Autodesk Inventor part; units mm, degrees
ref_plane "YZ Plane" through (0, 0, 0) normal (1, 0, 0) x (0, 1, 0)
ref_plane "XZ Plane" through (0, 0, 0) normal (0, 1, 0) x (-1, 0, 0)
ref_plane "XY Plane" through (0, 0, 0) normal (0, 0, 1) x (1, 0, 0)
sketch "Sketch1" plane through (0, 0, 0) normal (0, 1, 0) x (-1, 0, 0)
  circle A0 centre (0, 0) radius 4
  circle A1 centre (0, 0) radius 35
  circle A2 centre (0, -28) radius 2
  circle A3 centre (14, -24.2487) radius 2
  circle A4 centre (24.2487, -14) radius 2
  circle A5 centre (28, 0) radius 2
  circle A6 centre (24.2487, 14) radius 2
  circle A7 centre (14, 24.2487) radius 2
  circle A8 centre (0, 28) radius 2
  circle A9 centre (-14, 24.2487) radius 2
  circle A10 centre (-24.2487, 14) radius 2
  circle A11 centre (-28, 0) radius 2
  circle A12 centre (-24.2487, -14) radius 2
  circle A13 centre (-14, -24.2487) radius 2
  circle A14 centre (-12, 0) radius 2.05
  circle A15 centre (6, -10.3923) radius 2.05
  circle A16 centre (6, 10.3923) radius 2.05
  dimension "d0" = 70
  dimension "d1" = 8
  dimension "d4" = 4
  dimension "d5" = 28
  dimension "d8" = 360
  dimension "d21" = 14.4939
  dimension "d53" = 12
  dimension "d54" = 4.1
  dimension "d57" = 360
extrude "Extrusion1" add sketch "Sketch1" along normal blind 4 contours A1 | A2 | A3 | A4 | A5 | A6 | A7 | A8 | A9 | A10 | A11 | A12 | A13
chamfer "Chamfer2" distance 0.5 angle 45 4 edges at (35, 4, 0) (4, 4, 0) (35, 0, 0) (4, 0, 0)
chamfer "Chamfer3" distance 2.5 angle 45 3 edges at (-3.95, 4, 10.3923) (-3.95, 4, -10.3923) (14.05, 4, 0)
hole "Hole1" at (-24.2487, 0, -14) at (-28, 0, 0) at (-24.2487, 0, 14) at (-14, 0, 24.2487) at (0, 0, 28) at (14, 0, 24.2487) at (24.2487, 0, 14) at (28, 0, 0) at (24.2487, 0, -14) at (14, 0, -24.2487) at (0, 0, -28) at (-14, 0, -24.2487) direction (0, 1, 0) diameter 3.242 depth 15 tip angle 118
properties part number "end effector mount 4 mm" material "Aluminum 6061"
The model under review builds one solid part; all positions refer to its coordinate system, in mm. Coordinates: 2 decimals unless noted, no trailing zeros. Order: outer loops, then holes, each group sorted by start corner. A loop starts at its lowest first (then second) coordinate and runs counter-clockwise, first axis right, second up. Notation, with made-up numbers: (22.5, 0.25) -> (36.5, 0.25) arc R8 cw to (36.5, 4.25) -> close; hole circle Ø11 at (-34.5, -29). An arc over 180 degrees is marked (long way). Answer in a Markdown table with one row per item. Add a question column.
Item 1: Clearance check with flat-ended pins moving along their axes: pin 1 (1.9 mm diameter, centred on x = 0, z = 28, fed in from +Y); pin 2 (1.5 mm diameter, centred on y = 1, z = -15, fed in from -X); pin 3 (2 mm diameter, centred on x = -23.5, y = 1.5, fed in from +Z); pin 4 (1.5 mm diameter, centred on x = -3.5, y = 1, fed in from +Z). State where each tip first meets the part, or that it passes through.
Item 2: We need section A-A on z = 0. Give the number of separate pieces and of enclosed holes in the cut face, plus the area to 3 significant figures.
Item 3: We need section B-B on x = 0. Write out the cut boundary in (y, z), plus the area to 3 significant figures.
Item 4: Mouldability with a two-part tool opening along X and no side actions: class faces 1 (the cylindrical face through (13.513, 2.028, -25.795)), 2 (the flat face through (0, 0, -7)) as +X half, -X half, draft (parallel to the pull), parting line (faces both ways), or undercut.
Item 5: To check wall thickness, follow probe 1 along Z at (x, y) = (0, 3.4); probe 2 along Z at (x, y) = (-14, 1.6); probe 3 along Z at (x, y) = (-7, 0.95). State the ranges of each line that lie inside material, in increasing order.
Final values:
| question | item | result |
|---|---|---|
| 1 | pin 1 | passes through |
| 1 | pin 2 | stops at x = -31.97 |
| 1 | pin 3 | stops at z = 26.81 |
| 1 | pin 4 | stops at z = 34.89 |
| 2 | separate pieces | 5 |
| 2 | enclosed holes | 0 |
| 2 | area | 198 mm2 |
| 3 | outline | (0, -34.5) -> (0.5, -35) -> (3.5, -35) -> (4, -34.5) -> (4, -29.62) -> (0, -29.62) -> close; (0, -26.38) -> (4, -26.38) -> (4, -4.5) -> (3.5, -4) -> (0.5, -4) -> (0, -4.5) -> close; (0, 4.5) -> (0.5, 4) -> (3.5, 4) -> (4, 4.5) -> (4, 26.38) -> (0, 26.38) -> close; (0, 29.62) -> (4, 29.62) -> (4, 34.5) -> (3.5, 35) -> (0.5, 35) -> (0, 34.5) -> close |
| 3 | area | 221 mm2 |
| 4 | face 1 | undercut |
| 4 | face 2 | draft |
| 5 | probe 1 | z = -35 to -29.62, -26.38 to -4, 4 to 26.38, 29.62 to 35 |
| 5 | probe 2 | z = -32.08 to -25.87, -22.63 to 22.63, 25.87 to 32.08 |
| 5 | probe 3 | z = -34.29 to -12.18, -8.6 to 8.6, 12.18 to 34.29 |
